The listing builds one solid part. Answer for the finished solid, in the listing's coordinates (mm). Face numbers are marked on the shaded views. Coordinates: 2 decimals unless noted, no trailing zeros. Order: outer loops, then holes, each group sorted by start corner. A loop starts at its lowest first (then second) coordinate and runs counter-clockwise, first axis right, second up.
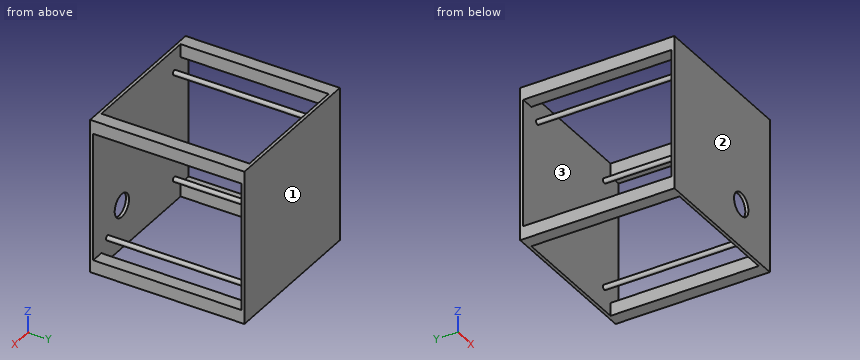
from build123d import *

# Parameters (mm, degrees)
SKETCH1_W            = 100
SKETCH1_H            = 100
BASE_DEPTH           = 2
SKETCH2_W            = 8.5
SKETCH2_H            = 8.5
BOSS_EXTRUDE2_DEPTH  = 96
LPATTERN1_COUNT      = 2
LPATTERN1_PITCH      = 91.5
LPATTERN1_COUNT_DIR2 = 2
LPATTERN1_PITCH_DIR2 = 91.5
LPATTERN2_COUNT      = 2
LPATTERN2_PITCH      = 98
SKETCH3_R            = 1.575
RODS_DEPTH           = 96
LPATTERN3_COUNT      = 2
LPATTERN3_PITCH      = 70
LPATTERN3_COUNT_DIR2 = 2
LPATTERN3_PITCH_DIR2 = 70
SKETCH5_R            = 7.5
CUT_EXTRUDE1_DEPTH   = 10


with BuildPart() as part:
    # Sketch1 → Base (new body)
    with BuildSketch(Plane(origin=(0, 0, 0), x_dir=(1, 0, 0), z_dir=(0, 1, 0))):
        with Locations((50, 50)):
            Rectangle(SKETCH1_W, SKETCH1_H)
    base = extrude(amount=BASE_DEPTH)

    # Sketch2 → Boss-Extrude2 (add)
    with BuildSketch(Plane(origin=(0, 2, 0), x_dir=(1, 0, 0), z_dir=(0, 1, 0))):
        with Locations((4.25, 4.25)):
            Rectangle(SKETCH2_W, SKETCH2_H)
    boss_extrude2 = extrude(amount=BOSS_EXTRUDE2_DEPTH)

    # LPattern1: Boss-Extrude2 2 × 2
    with Locations(*[(j * LPATTERN1_PITCH_DIR2, 0, -i * LPATTERN1_PITCH) for i in range(LPATTERN1_COUNT) for j in range(LPATTERN1_COUNT_DIR2) if (i, j) != (0, 0)]):
        add(boss_extrude2)

    # LPattern2: Base ×2
    with Locations(*[(0, i * LPATTERN2_PITCH, 0) for i in range(1, LPATTERN2_COUNT)]):
        add(base)

    # Sketch3 → Rods (add)
    with BuildSketch(Plane(origin=(0, 2, 0), x_dir=(1, 0, 0), z_dir=(0, 1, 0))):
        with Locations((15, 85)):
            Circle(SKETCH3_R)
    rods = extrude(amount=RODS_DEPTH)

    # LPattern3: Rods 2 × 2
    with Locations(*[(i * LPATTERN3_PITCH, 0, j * LPATTERN3_PITCH_DIR2) for i in range(LPATTERN3_COUNT) for j in range(LPATTERN3_COUNT_DIR2) if (i, j) != (0, 0)]):
        add(rods)

    # Sketch5 → Cut-Extrude1 (cut)
    with BuildSketch(Plane(origin=(0, 2, 0), x_dir=(1, 0, 0), z_dir=(0, 1, 0))):
        with Locations((70, 72)):
            Circle(SKETCH5_R)
    extrude(amount=-CUT_EXTRUDE1_DEPTH, mode=Mode.SUBTRACT)


solid = part.part
1) Consider L1, parallel to X at y = 0.7, z = -72; L2, parallel to Z at x = 70, y = 1.3; L3, parallel to Y at x = 35, z = -84. Determine where each line is inside the solid, lowest interval first.
2) Section B-B (y = 25) is taken. Give the vertices of the cut face in (x, z) (3 decimals).
3) Determine the mould class of the marked faces 1, 2 and 3 for opening direction Y: released by +Y, released by -Y, zero draft, split by the parting line, or undercut.
4) Section D-D (z = -19.5) is taken. Give the vertices of the cut face in (x, y).
5) This flat-tipped pin is pushed along its axis until it touches: P1, Ø10, axis at y = 62, z = -80, coming from the -X side (3 decimals). Where does it stop, or does it pass through?
6) Section A-A (x = 30) is taken. Give the vertices of the cut face in (y, z).
7) Section C-C (x = 70) is taken. Give the vertices of the cut face in (y, z), then the cut area to 3 significant figures.
Filled sheet:
1. L1: x = 0 to 62.5, 77.5 to 100
1. L2: z = -100 to -79.5, -64.5 to 0
1. L3: y = 0 to 2, 98 to 100
2. outline: (0, -100) - (8.5, -100) - (8.5, -91.5) - (0, -91.5) - close; (0, -8.5) - (8.5, -8.5) - (8.5, 0) - (0, 0) - close; circle Ø3.15 at (15, -85); circle Ø3.15 at (15, -15); circle Ø3.15 at (85, -85); circle Ø3.15 at (85, -15); (91.5, -100) - (100, -100) - (100, -91.5) - (91.5, -91.5) - close; (91.5, -8.5) - (100, -8.5) - (100, 0) - (91.5, 0) - close
3. face 1: released by +Y
3. face 2: released by -Y
3. face 3: undercut
4. outline: (0, 0) - (100, 0) - (100, 2) - (0, 2) - close; (0, 98) - (100, 98) - (100, 100) - (0, 100) - close
5. P1: stops at x = 13.425
6. outline: (0, -100) - (2, -100) - (2, 0) - (0, 0) - close; (98, -100) - (100, -100) - (100, 0) - (98, 0) - close
7. outline: (0, -100) - (2, -100) - (2, -79.5) - (0, -79.5) - close; (0, -64.5) - (2, -64.5) - (2, 0) - (0, 0) - close; (98, -100) - (100, -100) - (100, 0) - (98, 0) - close
7. area: 370 mm2
